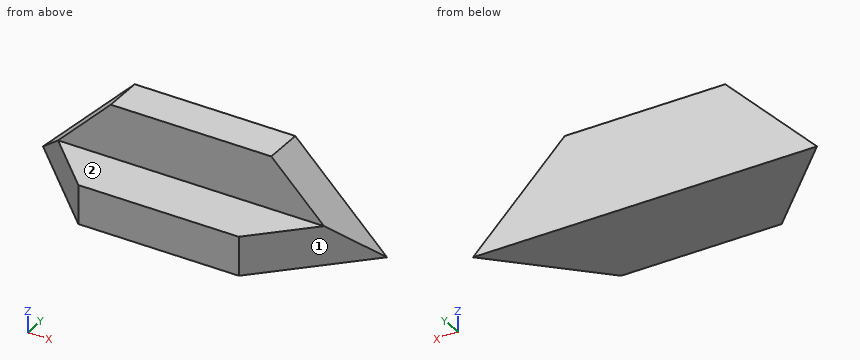
from build123d import *

# Parameters (mm, degrees)
BOSS_EXTRU_1_DEPTH      = 150
ENL_V_MAT_EXTRU_1_DEPTH = 41
ENL_V_MAT_EXTRU_2_DEPTH = 41


with BuildPart() as part:
    # Esquisse1 → Boss.-Extru.1 (new body)
    with BuildSketch(Plane(origin=(0, 0, 0), x_dir=(0, 0, -1), z_dir=(1, 0, 0))):
        Polygon((0, 0), (-40, 0), (-40, -17), (-17, -17), (-17, -40), (0, -40), align=None)
    extrude(amount=BOSS_EXTRU_1_DEPTH)

    # Esquisse2 → Enlèv. mat.-Extru.1 (cut, through all)
    with BuildSketch(Plane(origin=(0, 0, 0), x_dir=(1, 0, 0), z_dir=(0, 1, 0))):
        Polygon((150, 0), (110, -40), (150, -40), align=None)
        Polygon((0, 0), (0, -40), (40, -40), align=None)
    extrude(amount=-ENL_V_MAT_EXTRU_1_DEPTH, mode=Mode.SUBTRACT)

    # Esquisse3 → Enlèv. mat.-Extru.2 (cut, through all)
    with BuildSketch(Plane(origin=(0, 0, 0), x_dir=(-1, 0, 0), z_dir=(0, 0, -1))):
        Polygon((-150, 0), (-110, -40), (-150, -40), align=None)
        Polygon((-40, -40), (0, -40), (0, 0), align=None)
    extrude(amount=-ENL_V_MAT_EXTRU_2_DEPTH, mode=Mode.SUBTRACT)


solid = part.part
Model file for the job. Use its own axes, mm. Face numbers are marked on the shaded views. A direction names the side the tool comes from. Round coordinates to 2 decimals unless told otherwise and drop trailing zeros. Loops run counter-clockwise (first coordinate to the right, second up) from the corner with the lowest first, then second, coordinate; pieces in that order, holes last. Notation, with made-up numbers: (-14.75, 58.5) -> (24.25, 58.5) arc R29 ccw to (24.25, 97.5) -> close; hole circle Ø8 at (35.5, -4). An arc over 180 degrees is marked (long way). Answer as CSV lines item,"result". Start each with the question number.
1) Slice it at D-D (y = -26). List the corners of the cut face in (x, z).
2) Slice it at A-A (y = -10.5). List the corners of the cut face in (x, z), plus the area to 3 significant figures.
3) Slice it at C-C (x = 140.5). List the corners of the cut face in (y, z).
4) Slice it at B-B (z = 12). List the corners of the cut face in (x, y), plus the area to 3 significant figures.
5) Pin check, flat tips, straight feed: P1, Ø1.5, axis at y = -33, z = 19.5, coming from the +X side; P2, Ø7, axis at x = 98.5, z = 28, coming from the -Y side; P3, Ø11.5, axis at x = 50.5, y = -26, coming from the +Z side. Stop position of each tip, or through.
6) Tool access for the marked faces 1 and 2: list every direction of +Z, -Z, +X, -X, +Y, -Y with a clear straight run to the whole face (end or side of a thin tool).
7) Probe line 1 along Y through (x, z) = (113.5, 18); line 2 along Z through (x, y) = (133, -14); line 3 along X through (y, z) = (-8.5, 17). List the from-to ranges inside material, lowest first.
Filled in:
1,outline,"(26, 0) -> (124, 0) -> (124, 17) -> (26, 17) -> close"
2,outline,"(10.5, 0) -> (139.5, 0) -> (139.5, 10.5) -> (110, 40) -> (40, 40) -> (10.5, 10.5) -> close"
2,area,"4,290 mm2"
3,outline,"(-9.5, 0) -> (0, 0) -> (0, 9.5) -> (-9.5, 9.5) -> close"
4,outline,"(12, -12) -> (40, -40) -> (110, -40) -> (138, -12) -> (138, 0) -> (12, 0) -> close"
4,area,"4,260 mm2"
5,P1,"passes through"
5,P2,"stops at y = -17"
5,P3,"stops at z = 17"
6,face 1,"+Z, -Z, +X, -Y"
6,face 2,"+Z, +X, -X, -Y"
7,line 1,"y = -17 to 0"
7,line 2,"z = 0 to 17"
7,line 3,"x = 17 to 133"
